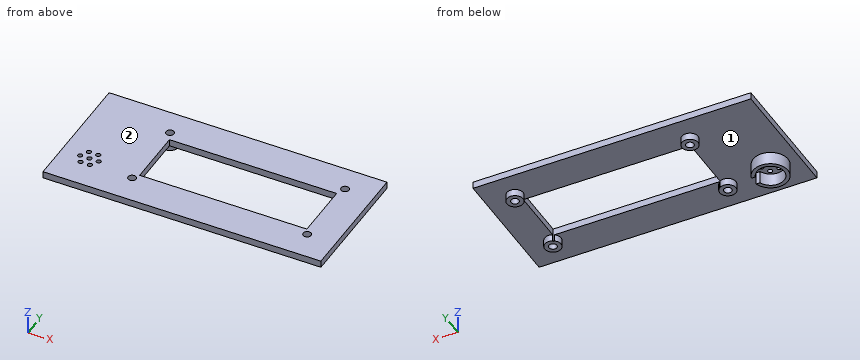
Autodesk Fusion 360 part; units mm, degrees
sketch "Sketch1" plane through (0, 0, 0) normal (0, 0, 1) x (1, 0, 0)
  line L0 (60, -27.5) -> (-60, -27.5)
  line L1 (-60, -27.5) -> (-60, 27.5)
  line L2 (-60, 27.5) -> (60, 27.5)
  line L3 (60, 27.5) -> (60, -27.5)
  line L4 (60, -27.5) -> (-60, 27.5) construction
  line L5 (-60, -27.5) -> (60, 27.5) construction
  dimension "d1" = 120
  dimension "d2" = 55
extrude "Extrude1" add sketch "Sketch1" along normal blind 3
sketch "Sketch2" plane through (0, 0, 3) normal (0, 0, 1) x (-1, 0, 0)
  line L0 (-60, -27.5) -> (60, -27.5)
  line L1 (60, -27.5) -> (60, 27.5)
  line L2 (60, 27.5) -> (-60, 27.5)
  line L3 (-60, 27.5) -> (-60, -27.5)
  line L4 (26.1, 12.4) -> (-46.1, 12.4)
  line L5 (-46.1, 12.4) -> (-46.1, -12.4)
  line L6 (-46.1, -12.4) -> (26.1, -12.4)
  line L7 (26.1, -12.4) -> (26.1, 12.4)
  line L8 (26.1, 12.4) -> (-46.1, -12.4) construction
  line L9 (-46.1, 12.4) -> (26.1, -12.4) construction
  point P0 (-10, 0)
  dimension "d5" = 72.2
  dimension "d6" = 24.8
extrude "Extrude2" cut sketch "Sketch2" against normal through all contours L4 L5 L6 L7
sketch "Sketch3" plane through (0, 0, 3) normal (0, 0, 1) x (-1, 0, 0)
  line L0 (26.1, -12.4) -> (-46.1, -12.4)
  line L1 (-46.1, -12.4) -> (-46.1, 12.4)
  line L2 (-46.1, 12.4) -> (26.1, 12.4)
  line L3 (26.1, 12.4) -> (26.1, -12.4)
  line L4 (-60, -27.5) -> (60, -27.5)
  line L5 (60, -27.5) -> (60, 27.5)
  line L6 (60, 27.5) -> (-60, 27.5)
  line L7 (-60, 27.5) -> (-60, -27.5)
  circle A0 centre (27.9, -16.35) radius 1.7
  circle A1 centre (-47.66, -16.35) radius 1.7
  circle A2 centre (27.9, 15.18) radius 1.7
  circle A3 centre (-47.66, 15.18) radius 1.7
  dimension "d9" = 3.4
  dimension "d10" = 27.9
  dimension "d11" = 16.35
  dimension "d14" = 75.56
  dimension "d15" = -31.53
extrude "Extrude3" cut sketch "Sketch3" against normal through all contours A0 | A1 | A2 | A3
sketch "Sketch5" plane through (0, 0, 3) normal (0, 0, 1) x (-1, 0, 0)
  circle A0 centre (-47.66, 15.18) radius 1.7
  circle A1 centre (27.9, 15.18) radius 1.7
  circle A2 centre (27.9, -16.35) radius 1.7
  circle A3 centre (-47.66, -16.35) radius 1.7
  line L0 (26.1, -12.4) -> (-46.1, -12.4)
  line L1 (-46.1, -12.4) -> (-46.1, 12.4)
  line L2 (-46.1, 12.4) -> (26.1, 12.4)
  line L3 (26.1, 12.4) -> (26.1, -12.4)
  line L4 (-60, -27.5) -> (60, -27.5)
  line L5 (60, -27.5) -> (60, 27.5)
  line L6 (60, 27.5) -> (-60, 27.5)
  line L7 (-60, 27.5) -> (-60, -27.5)
  line L8 (56.1021, -14.9687) -> (33, -15) construction
  line L9 (33, -15) -> (33.013, -24.5594) construction
  line L10 (33.013, -24.5594) -> (56.1151, -24.5281) construction
  line L11 (56.1151, -24.5281) -> (56.1021, -14.9687) construction
  dimension "d24" = 3.5
sketch "Sketch6" plane through (0, 0, 3) normal (0, 0, 1) x (-1, 0, 0)
  line L0 (-60, -27.5) -> (60, -27.5)
  line L1 (60, -27.5) -> (60, 27.5)
  line L2 (60, 27.5) -> (-60, 27.5)
  line L3 (-60, 27.5) -> (-60, -27.5)
  line L4 (26.1, -12.4) -> (-46.1, -12.4)
  line L5 (-46.1, -12.4) -> (-46.1, 12.4)
  line L6 (-46.1, 12.4) -> (26.1, 12.4)
  line L7 (26.1, 12.4) -> (26.1, -12.4)
  circle A0 centre (-47.66, -16.35) radius 1.7
  circle A1 centre (27.9, -16.35) radius 1.7
  circle A2 centre (27.9, 15.18) radius 1.7
  circle A3 centre (-47.66, 15.18) radius 1.7
  circle A4 centre (48, 12) radius 1
  circle A5 centre (44, 12) radius 1
  circle A6 centre (46, 8.5359) radius 1
  circle A7 centre (50, 8.5359) radius 1
  circle A8 centre (52, 12) radius 1
  circle A9 centre (50, 15.4641) radius 1
  circle A10 centre (46, 15.4641) radius 1
  dimension "d29" = 2
  dimension "d30" = 48
  dimension "d31" = 12
  dimension "d32" = 2
  dimension "d33" = 4
  dimension "d35" = 360
extrude "Extrude6" cut sketch "Sketch6" against normal through all contours A4 | A5 | A6 | A7 | A8 | A9 | A10
sketch "Sketch7" plane through (0, 0, 0) normal (0, 0, 1) x (1, 0, 0)
  arc A0 (-40.7716, -10) -> (-40.7716, -14) centre (-48, -12) ccw
  arc A1 (-42.4493, -10) -> (-42.4493, -14) centre (-48, -12) ccw
  line L0 (-40.7716, -10) -> (-42.4493, -10)
  line L1 (-40.7716, -14) -> (-42.4493, -14)
  dimension "d37" = 11.8
  dimension "d38" = 48
  dimension "d39" = 12
  dimension "d40" = 15
  dimension "d41" = 2
  dimension "d42" = 2
extrude "Extrude7" add sketch "Sketch7" against normal blind 5.5
sketch "Sketch8" plane through (0, 0, 0) normal (0, 0, -1) x (1, 0, 0)
  circle A0 centre (-46, 15.4641) radius 1
  circle A1 centre (-48, 12) radius 1
  circle A2 centre (-50, 15.4641) radius 1
  circle A3 centre (-44, 12) radius 1
  circle A4 centre (-50, 8.5359) radius 1
  circle A5 centre (-52, 12) radius 1
  circle A6 centre (-46, 8.5359) radius 1
  line L0 (-60, -27.5) -> (60, -27.5)
  line L1 (60, -27.5) -> (60, 27.5)
  line L2 (60, 27.5) -> (-60, 27.5)
  line L3 (-60, 27.5) -> (-60, -27.5)
  line L4 (46.1, -12.4) -> (-26.1, -12.4)
  line L5 (-26.1, -12.4) -> (-26.1, 12.4)
  line L6 (-26.1, 12.4) -> (46.1, 12.4)
  line L7 (46.1, 12.4) -> (46.1, -12.4)
  circle A7 centre (47.66, -16.35) radius 1.7
  circle A8 centre (-27.9, -16.35) radius 1.7
  circle A9 centre (-27.9, 15.18) radius 1.7
  circle A10 centre (47.66, 15.18) radius 1.7
  line L8 (-40.7716, 14) -> (-42.4493, 14)
  arc A11 (-42.4493, 14) -> (-42.4493, 10) centre (-48, 12) ccw
  line L9 (-42.4493, 10) -> (-40.7716, 10)
  arc A12 (-40.7716, 14) -> (-40.7716, 10) centre (-48, 12) ccw
  circle A13 centre (47.66, -16.35) radius 1.7
  circle A14 centre (-27.9, -16.35) radius 1.7
  circle A15 centre (-27.9, 15.18) radius 1.7
  circle A16 centre (47.66, 15.18) radius 1.7
  circle A17 centre (47.66, -16.35) radius 3.5
  circle A18 centre (-27.9, -16.35) radius 3.5
  arc A19 (46.1, 12.0469) -> (45.5336, 12.4) centre (47.66, 15.18) ccw
  arc A20 (-25.7736, 12.4) -> (-26.1, 12.1783) centre (-27.9, 15.18) ccw
  point P0 (46.1, 12.4)
  point P1 (46.1, -12.4)
  point P2 (-26.1, -12.4)
  point P3 (-26.1, 12.4)
  dimension "d45" = 7
  dimension "d46" = 7
  dimension "d47" = 7
  dimension "d48" = 7
extrude "Extrude8" add sketch "Sketch8" along normal blind 3 contours L6 L7 A19 | L5 L6 A20 | A17 | A18
Read the model definition and answer for the solid it produces. Units are mm, in the model's axes. Face numbers are marked on the shaded views. Give positions to 0.01 mm unless a question says otherwise; leave off trailing zeros. Order: outer loops, then holes, each group sorted by start corner. A loop starts at its lowest first (then second) coordinate and runs counter-clockwise, first axis right, second up. Notation, with made-up numbers: (7, 43.25) -> (17, 43.25) arc R25 ccw to (17, 60.25) -> close; hole circle Ø8 at (31, -6.5). An arc over 180 degrees is marked (long way). One line per item, written item: value. Start each with the question number.
(1) The part is cut by section B-B (x = 8). Determine the outline of the cut face in (y, z), and give its area (3 significant figures).
(2) For a pull along X with two mould halves and no side action, classify the marked faces 1 and 2 as released by +X, released by -X, zero draft, split by the parting line, or undercut.
(3) The part is cut by section C-C (y = 16.35). Determine the outline of the cut face in (x, z), and give its area (3 significant figures).
(4) The part is cut by section D-D (z = -1.25). State how many separate pieces and enclosed holes the cut face has, and give its area (3 significant figures).
(5) Straight lines are drawn through the part: L1, parallel to Y at x = -27.9, z = -2.4; L2, parallel to X at y = 16.35, z = 1.4; L3, parallel to X at y = 16.35, z = -1.45. For each, find the intervals that lie inside material, in ascending order.
(6) The part is cut by section A-A (y = -2.5). Determine the outline of the cut face in (x, z), and give its area (3 significant figures).
(7) Flat-ended cylindrical pins translate along their axes: P1, Ø16.5, axis at x = 8, y = 9.5, coming from the -Z side; P2, Ø3, axis at x = -44, y = -12, coming from the +Z side; P3, Ø3.5, axis at x = -27, y = 15, coming from the -Z side; P4, Ø1.8, axis at x = -42, z = -3.5, coming from the +Y side. Find the tip coordinate at first contact, or state that the pin passes through.
Taken from the geometry:
1. outline: (-27.5, 0) -> (-12.4, 0) -> (-12.4, 3) -> (-27.5, 3) -> close; (12.4, 0) -> (27.5, 0) -> (27.5, 3) -> (12.4, 3) -> close
1. area: 90.6 mm^2
2. face 1: undercut
2. face 2: zero draft
3. outline: (-60, 0) -> (-31.4, 0) -> (-31.4, -3) -> (-29.6, -3) -> (-29.6, 3) -> (-60, 3) -> close; (-26.2, -3) -> (-24.4, -3) -> (-24.4, 0) -> (44.16, 0) -> (44.16, -3) -> (45.96, -3) -> (45.96, 3) -> (-26.2, 3) -> close; (49.36, -3) -> (51.16, -3) -> (51.16, 0) -> (60, 0) -> (60, 3) -> (49.36, 3) -> close
3. area: 361 mm^2
4. separate pieces: 5
4. enclosed holes: 4
4. area: 178 mm^2
5. L1: -18.68 to -16.88, -13.48 to -11.68, 12.85 to 14.65, 18.05 to 19.85
5. L2: -60 to -29.6, -26.2 to 45.96, 49.36 to 60
5. L3: -31.4 to -29.6, -26.2 to -24.4, 44.16 to 45.96, 49.36 to 51.16
6. outline: (-60, 0) -> (-26.1, 0) -> (-26.1, 3) -> (-60, 3) -> close; (46.1, 0) -> (60, 0) -> (60, 3) -> (46.1, 3) -> close
6. area: 143 mm^2
7. P1: z = 0
7. P2: z = 3
7. P3: z = -3
7. P4: y = -6.5
